Work out the finished part from the listing and answer in its coordinate system (mm). Face numbers are marked on the shaded views. A direction names the side the tool comes from. Coordinates: 2 decimals unless noted, no trailing zeros. Order: outer loops, then holes, each group sorted by start corner. A loop starts at its lowest first (then second) coordinate and runs counter-clockwise, first axis right, second up. Notation, with made-up numbers: (22.5, 49) -> (32.5, 49) arc R12 ccw to (32.5, 55) -> close; hole circle Ø11 at (62.25, 35.5). An arc over 180 degrees is marked (long way). Write item = value, one per line. Start each with the question number.
Q1. Straight lines are drawn through the part: L1, parallel to X at y = -0.5, z = 2.25; L2, parallel to X at y = 2.25, z = 1.4; L3, parallel to Y at x = 18.85, z = 2. For each, find the intervals that lie inside material, in ascending order. Write a range as from..to.
Q2. The part is cut by section B-B, the plane y = 0. Determine the outline of the cut face in (x, z), plus the area to 3 significant figures.
Q3. The part is cut by section D-D, the plane y = 1.25. Determine the outline of the cut face in (x, z).
Q4. For a pull along Y with two mould halves and no side action, classify the marked faces 4, 5 and 6 as +Y half, -Y half, draft (parallel to the pull), parting line (faces both ways), or undercut.
Q5. Flat-ended cylindrical pins translate along their axes: pin 1 (1.6 mm diameter, centred on x = 14.5, z = 1.5, fed in from -Y); pin 2 (1.5 mm diameter, centred on x = 7.5, z = 2, fed in from -Y); pin 3 (1.5 mm diameter, centred on x = 11, z = 1, fed in from +Y). Find the tip coordinate at first contact, or state that the pin passes through.
Q6. The part is cut by section A-A, the plane z = 2.3. Determine the outline of the cut face in (x, y), plus the area to 3 significant figures.
Q7. Which of the six approach directions +Z, -Z, +X, -X, +Y, -Y give full straight-line access (tool end or side, diameter ignored) to the marked faces 1, 2 and 3?
Q8. The part is cut by section C-C, the plane x = -1.25. Determine the outline of the cut face in (y, z).
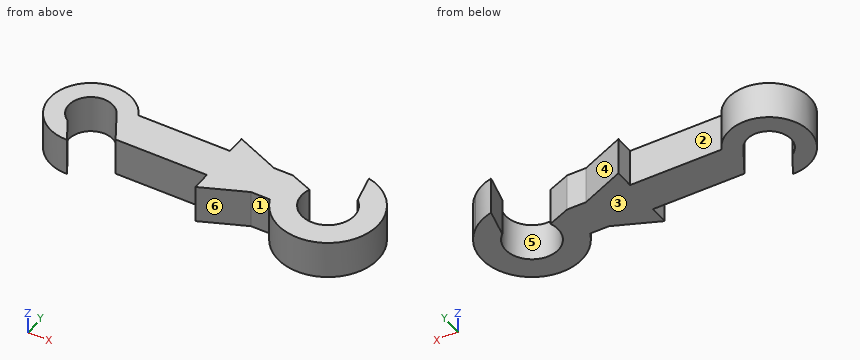
```python
from build123d import *

# Parameters (mm, degrees)
PAD_DEPTH = 3


with BuildPart() as part:
    # Sketch → Pad (new body)
    with BuildSketch(Plane.XY):
        with BuildLine():
            ThreePointArc((15.141901, -1.5), (21.144306, -3.276608), (21.527784, 2.971443))
            ThreePointArc((21.527784, 2.971443), (20.682106, 3.555754), (19.715442, 3.905254))
            Line((20.255836, 1.560008), (19.715442, 3.905254))
            ThreePointArc((16.903248, 0.7875), (19.321529, -2.046377), (20.255836, 1.560008))
            Line((16.903248, 0.7875), (15.141901, 1.5))
            Line((15.141901, 1.5), (13.641901, 1.5))
            Line((13.641901, 1.5), (10.141901, 3))
            Line((10.141901, 3), (10.141901, 1.5))
            Line((10.141901, 1.5), (2.883141, 1.5))
            ThreePointArc((2.883141, 1.5), (-2.8, 1.65), (0.084684, -3.248897))
            Line((0.084684, -3.248897), (-0.938159, -1.47728))
            ThreePointArc((1.460552, 0.963995), (-1.248271, 1.226507), (-0.938159, -1.47728))
            Line((2.883141, -1.5), (1.460552, 0.963995))
            Line((10.141901, -1.5), (2.883141, -1.5))
            Line((10.141901, -3), (10.141901, -1.5))
            Line((13.641901, -1.5), (10.141901, -3))
            Line((15.141901, -1.5), (13.641901, -1.5))
        make_face()
    extrude(amount=PAD_DEPTH)


solid = part.part
```
Model answer:
q1.L1 = -3.21..-1.68, 2.31..16.81, 20.89..22.82
q1.L2 = -2.35..2.35, 10.14..11.89, 20.1..22.16
q1.L3 = -4..-2.1
q2.outline = (-3.25, 0) -> (-1.75, 0) -> (-1.75, 3) -> (-3.25, 3) -> close; (2.02, 0) -> (16.75, 0) -> (16.75, 3) -> (2.02, 3) -> close; (20.95, 0) -> (22.85, 0) -> (22.85, 3) -> (20.95, 3) -> close
q2.area = 54.4 mm2
q3.outline = (-3, 0) -> (-1.22, 0) -> (-1.22, 3) -> (-3, 3) -> close; (1.22, 0) -> (15.76, 0) -> (15.76, 3) -> (1.22, 3) -> close; (20.54, 0) -> (22.65, 0) -> (22.65, 3) -> (20.54, 3) -> close
q4.face_4 = +Y half
q4.face_5 = undercut
q4.face_6 = -Y half
q5.pin_1 = -1.84
q5.pin_2 = -1.5
q5.pin_3 = 2.95
q6.outline = (-0.94, -1.48) arc R1.75 cw (long way) to (1.46, 0.96) -> (2.88, -1.5) -> (10.14, -1.5) -> (10.14, -3) -> (13.64, -1.5) -> (15.14, -1.5) arc R4 ccw (long way) to (21.53, 2.97) arc R4 ccw to (19.72, 3.91) -> (20.26, 1.56) arc R2.1 cw (long way) to (16.9, 0.79) -> (15.14, 1.5) -> (13.64, 1.5) -> (10.14, 3) -> (10.14, 1.5) -> (2.88, 1.5) arc R3.25 ccw (long way) to (0.08, -3.25) -> close
q6.area = 86.1 mm2
q7.face_1 = +Z, -Z, -Y
q7.face_2 = +Z, -Z, +Y
q7.face_3 = -Z, +X, -X, +Y, -Y
q8.outline = (-3, 0) -> (-1.22, 0) -> (-1.22, 3) -> (-3, 3) -> close; (1.22, 0) -> (3, 0) -> (3, 3) -> (1.22, 3) -> close
